Check sheet for the modelled part. Datum: model origin and axes. Units: mm. Face numbers are marked on the shaded views. A direction names the side the tool comes from. Give positions to 0.01 mm unless a question says otherwise; leave off trailing zeros. Write each loop counter-clockwise with the first axis right and the second up, starting at its lowest first coordinate (ties: lowest second). Pieces come first, ordered by that corner, then holes. Notation, with made-up numbers: (64, 59.5) -> (104, 59.5) arc R16 ccw to (104, 86.5) -> close; hole circle Ø10 at (26, 86). An arc over 180 degrees is marked (long way). Use a Markdown table: item, result. Add a question column.
1. Set-up check for the marked faces 4, 5 and 6: record each of +Z, -Z, +X, -X, +Y, -Y from which the full face is reachable in a straight line by a thin tool's end or side.
2. Scan lines: probe 1 along Z at (x, y) = (-4.5, 7.5); probe 2 along X at (y, z) = (3, -9.5); probe 3 along X at (y, z) = (5.25, -5.25). Record each from-to range of solid material in increasing order. Write a range as [from, to].
3. Cross-section at C-C (y = 0.5). Enter the section's corners in (x, z), then the cut area to 3 significant figures.
4. Release check for a two-part mould opening along Z. For the marked faces 1, 2 and 3 record: released by +Z, released by -Z, zero draft, split by the parting line, or undercut.
5. Gauge pin test, flat ends, axial feed: P1, Ø4, axis at y = 6.5, z = -4.5, coming from the +X side; P2, Ø6.5, axis at x = -2.5, y = 4, coming from the +Z side; P3, Ø1.6, axis at y = 6, z = -3, coming from the -X side. Record the tip position at first contact, or that the pin passes through.
6. Cross-section at D-D (z = -2). Enter the section's corners in (x, y).
7. Cross-section at A-A (z = -12.75). Enter the section's corners in (x, y), then the cut area to 3 significant figures.
8. Cross-section at B-B (x = -2). Enter the section's corners in (y, z), then the cut area to 3 significant figures.
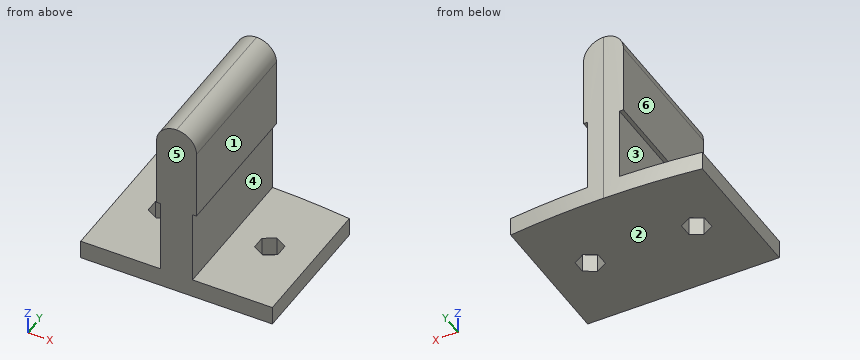
from build123d import *

# Parameters (mm, degrees)
BOSS_EXTRUDE1_DEPTH = 11
CUT_EXTRUDE1_DEPTH  = 20.949937343
CUT_EXTRUDE2_DEPTH  = 19.601075238
CUT_EXTRUDE3_DEPTH  = 20.949937343
CUT_EXTRUDE4_DEPTH  = 20.949937514


with BuildPart() as part:
    # Sketch1 → Boss-Extrude1 (new body)
    with BuildSketch(Plane(origin=(0, 0, 0), x_dir=(1, 0, 0), z_dir=(0, 1, 0))):
        Polygon((0, 0), (0, 12), (-6, 12), (-6, 14), (9, 14), (9, 12), (3, 12), (3, 0), align=None)
    extrude(amount=BOSS_EXTRUDE1_DEPTH)

    # Sketch3 → Cut-Extrude1 (cut, through all)
    with BuildSketch(Plane(origin=(0, 0, -14), x_dir=(-1, 0, 0), z_dir=(0, 0, -1))):
        with BuildLine():
            Line((-9, 11), (-9, 10.529404499))
            ThreePointArc((-9, 10.529404499), (-5.257374753, 10.882235554), (-1.5, 11))
            Line((-1.5, 11), (-9, 11))
        make_face()
        with BuildLine():
            Line((6, 11), (-1.5, 11))
            ThreePointArc((-1.5, 11), (2.257374753, 10.882235554), (6, 10.529404499))
            Line((6, 10.529404499), (6, 11))
        make_face()
    extrude(amount=-CUT_EXTRUDE1_DEPTH, mode=Mode.SUBTRACT)

    # Sketch4 → Cut-Extrude2 (cut, through all)
    with BuildSketch(Plane.XY.offset(-12)):
        Polygon((-2.5, 6.5), (-3.366025404, 6), (-3.366025404, 5), (-2.5, 4.5), (-1.633974596, 5), (-1.633974596, 6), align=None)
        Polygon((5.5, 6.5), (4.633974596, 6), (4.633974596, 5), (5.5, 4.5), (6.366025404, 5), (6.366025404, 6), align=None)
    extrude(amount=-CUT_EXTRUDE2_DEPTH, mode=Mode.SUBTRACT)

    # Sketch7 → Cut-Extrude3 (cut, through all)
    with BuildSketch(Plane.XZ):
        with BuildLine():
            ThreePointArc((0, -1.5), (0.439339828, -0.439339828), (1.5, 0))
            Line((1.5, 0), (0, 0))
            Line((0, 0), (0, -1.5))
        make_face()
        with BuildLine():
            Line((3, -1.5), (3, 0))
            Line((3, 0), (1.5, 0))
            ThreePointArc((1.5, 0), (2.560660172, -0.439339828), (3, -1.5))
        make_face()
    extrude(amount=-CUT_EXTRUDE3_DEPTH, mode=Mode.SUBTRACT)

    # Sketch8 → Cut-Extrude4 (cut, through all)
    with BuildSketch(Plane.XZ):
        Polygon((0.3, -6.75), (0, -6.75), (0, -12), (-6, -12), (-6, -14), (9, -14), (9, -12), (3, -12), (3, -6.75), (2.7, -6.75), (2.7, -12.3), (8.7, -12.3), (8.7, -13.7), (-5.7, -13.7), (-5.7, -12.3), (0.3, -12.3), align=None)
    extrude(amount=-CUT_EXTRUDE4_DEPTH, mode=Mode.SUBTRACT)


solid = part.part
Worked answers:
| question | item | result |
|---|---|---|
| 1 | face 4 | +X, +Y, -Y |
| 1 | face 5 | +Z, -Z, +X, -X, -Y |
| 1 | face 6 | +Z, -X, +Y, -Y |
| 2 | probe 1 | z = [-13.7, -12.3] |
| 2 | probe 2 | x = [0.3, 2.7] |
| 2 | probe 3 | x = [0, 3] |
| 3 | outline | (-5.7, -13.7) -> (8.7, -13.7) -> (8.7, -12.3) -> (2.7, -12.3) -> (2.7, -6.75) -> (3, -6.75) -> (3, -1.5) arc R1.5 ccw to (0, -1.5) -> (0, -6.75) -> (0.3, -6.75) -> (0.3, -12.3) -> (-5.7, -12.3) -> close |
| 3 | area | 52.8 mm² |
| 4 | face 1 | zero draft |
| 4 | face 2 | released by -Z |
| 4 | face 3 | undercut |
| 5 | P1 | stops at x = 3 |
| 5 | P2 | stops at z = -0.2 |
| 5 | P3 | stops at x = 0 |
| 6 | outline | (0, 0) -> (3, 0) -> (3, 10.98) arc R60 ccw to (0, 10.98) -> close |
| 7 | outline | (-5.7, 0) -> (8.7, 0) -> (8.7, 10.57) arc R60 ccw to (-5.7, 10.57) -> close; hole (-3.37, 5) -> (-2.5, 4.5) -> (-1.63, 5) -> (-1.63, 6) -> (-2.5, 6.5) -> (-3.37, 6) -> close; hole (4.63, 5) -> (5.5, 4.5) -> (6.37, 5) -> (6.37, 6) -> (5.5, 6.5) -> (4.63, 6) -> close |
| 7 | area | 151 mm² |
| 8 | outline | (0, -13.7) -> (4.79, -13.7) -> (4.79, -12.3) -> (0, -12.3) -> close; (6.21, -13.7) -> (10.9, -13.7) -> (10.9, -12.3) -> (6.21, -12.3) -> close |
| 8 | area | 13.3 mm² |
